Read the model definition and answer for the solid it produces. Units are mm, in the model's axes. Face numbers are marked on the shaded views. A direction names the side the tool comes from. Give positions to 0.01 mm unless a question says otherwise; leave off trailing zeros. Loops run counter-clockwise (first coordinate to the right, second up) from the corner with the lowest first, then second, coordinate; pieces in that order, holes last. Notation, with made-up numbers: (-14.75, 65.25) - (43.25, 65.25) arc R8 ccw to (43.25, 75.25) - close; hole circle Ø10 at (0, 47.25). An arc over 180 degrees is marked (long way). Write item = value, one per line.
```python
from build123d import *

# Parameters (mm, degrees)
SKETCH_3_W                         = 8
SKETCH_3_H                         = 10
SM_BASE_FLANGE_1_DEPTH             = 1
SM_EDGE_FLANGE_1_STRIP_W           = 6
SM_EDGE_FLANGE_1_STRIP_H           = 1
SM_EDGE_FLANGE_1_STRIP_CUT_DEPTH   = 8
SM_EDGE_FLANGE_1_STRIP_2_W         = 6
SM_EDGE_FLANGE_1_STRIP_2_H         = 1
SM_EDGE_FLANGE_1_STRIP_CUT_2_DEPTH = 8
SM_EDGE_FLANGE_1_DEPTH             = 8
SM_EDGE_FLANGE_1_BEND_DEPTH        = 8
SM_EDGE_FLANGE_2_STRIP_W           = 6
SM_EDGE_FLANGE_2_STRIP_H           = 1
SM_EDGE_FLANGE_2_STRIP_CUT_DEPTH   = 8
SM_EDGE_FLANGE_2_DEPTH             = 8
SM_EDGE_FLANGE_3_STRIP_W           = 6
SM_EDGE_FLANGE_3_STRIP_H           = 1
SM_EDGE_FLANGE_3_STRIP_CUT_DEPTH   = 8
SM_EDGE_FLANGE_3_DEPTH             = 8
FILLET_1_R                         = 2
HOLE_WIZARD_4_0_4_1_D              = 4


# Sheet-metal steps are written as plain solids
with BuildPart() as part:
    # 草图3 → 基体-法兰1 (new body)
    with BuildSketch(Plane.XY.offset(15)):
        with Locations((62.047155018, 0)):
            Rectangle(SKETCH_3_W, SKETCH_3_H)
    extrude(amount=-SM_BASE_FLANGE_1_DEPTH)

    # 边线-法兰1 strip (across the edge) → 边线-法兰1 strip cut (cut)
    with BuildSketch(Plane(origin=(66.047155018, -5, 14), x_dir=(0, 1, 0), z_dir=(-1, 0, 0))):
        with Locations((-2, -0.5)):
            Rectangle(SM_EDGE_FLANGE_1_STRIP_W, SM_EDGE_FLANGE_1_STRIP_H)
    extrude(amount=SM_EDGE_FLANGE_1_STRIP_CUT_DEPTH, mode=Mode.SUBTRACT)

    # 边线-法兰1 strip 2 (across the edge) → 边线-法兰1 strip cut 2 (cut)
    with BuildSketch(Plane(origin=(58.047155018, 5, 14), x_dir=(0, -1, 0), z_dir=(1, 0, 0))):
        with Locations((-2, -0.5)):
            Rectangle(SM_EDGE_FLANGE_1_STRIP_2_W, SM_EDGE_FLANGE_1_STRIP_2_H)
    extrude(amount=SM_EDGE_FLANGE_1_STRIP_CUT_2_DEPTH, mode=Mode.SUBTRACT)

    # 边线-法兰1 section (across the edge) → 边线-法兰1 (add)
    with BuildSketch(Plane(origin=(66.047155018, -5, 14), x_dir=(0, 1, 0), z_dir=(-1, 0, 0))):
        with BuildLine():
            Line((-1, 1), (-1, 9))
            Line((-1, 9), (0, 9))
            Line((0, 9), (0, 1))
            ThreePointArc((0, 1), (0.292893219, 0.292893219), (1, 0))
            Line((1, 0), (1, -1))
            ThreePointArc((1, -1), (-0.414213562, -0.414213562), (-1, 1))
        make_face()
    extrude(amount=SM_EDGE_FLANGE_1_DEPTH)

    # 边线-法兰1 section 2 (across the edge) → 边线-法兰1 bend (add)
    with BuildSketch(Plane(origin=(58.047155018, 5, 14), x_dir=(0, -1, 0), z_dir=(1, 0, 0))):
        with BuildLine():
            Line((-1, 1), (-1, 9))
            Line((-1, 9), (0, 9))
            Line((0, 9), (0, 1))
            ThreePointArc((0, 1), (0.292893219, 0.292893219), (1, 0))
            Line((1, 0), (1, -1))
            ThreePointArc((1, -1), (-0.414213562, -0.414213562), (-1, 1))
        make_face()
    extrude(amount=SM_EDGE_FLANGE_1_BEND_DEPTH)

    # 边线-法兰2 strip (across the edge) → 边线-法兰2 strip cut (cut)
    with BuildSketch(Plane(origin=(58.047155018, -6, 5), x_dir=(0, 0, 1), z_dir=(1, 0, 0))):
        with Locations((-2, -0.5)):
            Rectangle(SM_EDGE_FLANGE_2_STRIP_W, SM_EDGE_FLANGE_2_STRIP_H)
    extrude(amount=SM_EDGE_FLANGE_2_STRIP_CUT_DEPTH, mode=Mode.SUBTRACT)

    # 边线-法兰2 section (across the edge) → 边线-法兰2 (add)
    with BuildSketch(Plane(origin=(58.047155018, -6, 5), x_dir=(0, 0, 1), z_dir=(1, 0, 0))):
        with BuildLine():
            Line((-1, 1), (-1, 11))
            Line((-1, 11), (0, 11))
            Line((0, 11), (0, 1))
            ThreePointArc((0, 1), (0.292893219, 0.292893219), (1, 0))
            Line((1, 0), (1, -1))
            ThreePointArc((1, -1), (-0.414213562, -0.414213562), (-1, 1))
        make_face()
    extrude(amount=SM_EDGE_FLANGE_2_DEPTH)

    # 边线-法兰3 strip (across the edge) → 边线-法兰3 strip cut (cut)
    with BuildSketch(Plane(origin=(66.047155018, 6, 5), x_dir=(0, 0, 1), z_dir=(-1, 0, 0))):
        with Locations((-2, -0.5)):
            Rectangle(SM_EDGE_FLANGE_3_STRIP_W, SM_EDGE_FLANGE_3_STRIP_H)
    extrude(amount=SM_EDGE_FLANGE_3_STRIP_CUT_DEPTH, mode=Mode.SUBTRACT)

    # 边线-法兰3 section (across the edge) → 边线-法兰3 (add)
    with BuildSketch(Plane(origin=(66.047155018, 6, 5), x_dir=(0, 0, 1), z_dir=(-1, 0, 0))):
        with BuildLine():
            Line((-1, 1), (-1, 11))
            Line((-1, 11), (0, 11))
            Line((0, 11), (0, 1))
            ThreePointArc((0, 1), (0.292893219, 0.292893219), (1, 0))
            Line((1, 0), (1, -1))
            ThreePointArc((1, -1), (-0.414213562, -0.414213562), (-1, 1))
        make_face()
    extrude(amount=SM_EDGE_FLANGE_3_DEPTH)

    # 圆角1
    fillet_1_edges = [part.edges().sort_by_distance(p)[0] for p in [
        (58.047155018, -17, 4.5),
        (66.047155018, -17, 4.5),
        (66.047155018, 17, 4.5),
        (58.047155018, 17, 4.5),
    ]]
    fillet(fillet_1_edges, radius=FILLET_1_R)

    # Ø4.0 (4) 直径孔1 (through all)
    with Locations(Plane.XY.offset(5)):
        with Locations((62.047155018, 12.5), (62.047155018, -12.5)):
            Hole(HOLE_WIZARD_4_0_4_1_D / 2)


solid = part.part
```
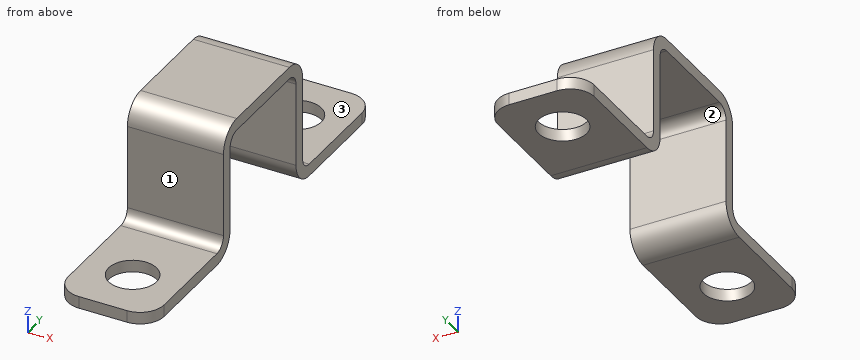
1) A cutting plane is placed at B-B on y = 12.5. Determine the outline of the cut face in (x, z).
Output:
outline = (58.05, 4) - (60.05, 4) - (60.05, 5) - (58.05, 5) - close; (64.05, 4) - (66.05, 4) - (66.05, 5) - (64.05, 5) - close
2) A cutting plane is placed at A-A on z = 7.5. Determine the outline of the cut face in (x, y), then the cut area to 3 significant figures.
Output:
outline = (58.05, -6) - (66.05, -6) - (66.05, -5) - (58.05, -5) - close; (58.05, 5) - (66.05, 5) - (66.05, 6) - (58.05, 6) - close
area = 16.0 mm²
3) A cutting plane is placed at D-D on x = 64.75. Determine the outline of the cut face in (y, z).
Output:
outline = (-16.87, 4) - (-7, 4) arc R2 ccw to (-5, 6) - (-5, 13) arc R1 cw to (-4, 14) - (4, 14) arc R1 cw to (5, 13) - (5, 6) arc R2 ccw to (7, 4) - (16.87, 4) - (16.87, 5) - (7, 5) arc R1 cw to (6, 6) - (6, 13) arc R2 ccw to (4, 15) - (-4, 15) arc R2 ccw to (-6, 13) - (-6, 6) arc R1 cw to (-7, 5) - (-16.87, 5) - close
4) Find the intervals of material crossed by probe 1 along Y at (x, z) = (63.25, 6.75); probe 2 along Z at (x, y) = (59.25, 11); probe 3 along Z at (x, y) = (62.5, -3), in increasing order.
Output:
probe_1 = -6 to -5, 5 to 6
probe_2 = 4 to 5
probe_3 = 14 to 15
5) A tool of negligible diameter and unlimited length cuts with its end or side. For the marked faces 1, 2 and 3, from which of +Z, -Z, +X, -X, +Y, -Y can it reach the whole face along a straight path? Write none if from no direction.
Output:
face_1 = +Z, +X, -X, -Y
face_2 = -Z, +X, -X
face_3 = +Z, +X, -X, +Y
6) Each of these flat-tipped pins is pushed along its axis until it touches: P1, Ø2.5, axis at x = 62, y = -1.5, coming from the -Z side; P2, Ø3, axis at x = 62.5, z = 14, coming from the +Y side. Where does it stop, or does it pass through?
Output:
P1 = 14
P2 = 6
7) A cutting plane is placed at C-C on x = 63.25. Determine the outline of the cut face in (y, z), then the cut area to 3 significant figures.
Output:
outline = (-17, 4) - (-14.1, 4) - (-14.1, 5) - (-17, 5) - close; (-10.9, 4) - (-7, 4) arc R2 ccw to (-5, 6) - (-5, 13) arc R1 cw to (-4, 14) - (4, 14) arc R1 cw to (5, 13) - (5, 6) arc R2 ccw to (7, 4) - (10.9, 4) - (10.9, 5) - (7, 5) arc R1 cw to (6, 6) - (6, 13) arc R2 ccw to (4, 15) - (-4, 15) arc R2 ccw to (-6, 13) - (-6, 6) arc R1 cw to (-7, 5) - (-10.9, 5) - close; (14.1, 4) - (17, 4) - (17, 5) - (14.1, 5) - close
area = 45.0 mm²
